Here's how the part is built. I have some questions about the finished solid (model axes, mm). A direction names the side the tool comes from. Round coordinates to 2 decimals unless told otherwise and drop trailing zeros. Write each loop counter-clockwise with the first axis right and the second up, starting at its lowest first coordinate (ties: lowest second). Pieces come first, ordered by that corner, then holes. Notation, with made-up numbers: (4.5, 50) - (35.5, 50) arc R15 cw to (35.5, 64) - close; hole circle Ø9 at (-3, 45). An arc over 180 degrees is marked (long way). Return JSON: item names as keys, results as strings. Group by question number.
```python
from build123d import *

# Parameters (mm, degrees)
SKETCH1_W               = 100
SKETCH1_H               = 45
BOSS_EXTRUDE1_DEPTH     = 90
CUT_EXTRUDE1_DEPTH      = 137.404728657
CUT_EXTRUDE2_DEPTH      = 109.397416943
CUT_EXTRUDE2_DEPTH_BACK = 109.397416943
SKETCH3_W               = 96
SKETCH3_H               = 32.638698082
SKETCH4_W               = 96
SKETCH4_H               = 35
CUT_EXTRUDE4_DEPTH      = 102.149641621
SKETCH5_R               = 8
SKETCH5_R_2             = 3
CUT_EXTRUDE5_DEPTH      = 134.158739856
SKETCH7_W               = 96
SKETCH7_H               = 3
CUT_EXTRUDE7_DEPTH      = 73.452349302
SKETCH9_W               = 50
SKETCH9_H               = 59.094844588
CUT_EXTRUDE9_DEPTH      = 34
SKETCH10_R              = 2
CUT_EXTRUDE10_DEPTH     = 34
CUT_EXTRUDE11_DEPTH     = 109.397416943
SKETCH11_W              = 96
SKETCH11_H              = 6.475085822
CUT_EXTRUDE12_DEPTH     = 34
SKETCH12_W              = 23
SKETCH12_H              = 26.924334535
CUT_EXTRUDE13_DEPTH     = 34


with BuildPart() as part:
    # Sketch1 → Boss-Extrude1 (new body)
    with BuildSketch(Plane.XY):
        Rectangle(SKETCH1_W, SKETCH1_H)
    extrude(amount=BOSS_EXTRUDE1_DEPTH)

    # Sketch2 → Cut-Extrude1 (cut, through all)
    with BuildSketch(Plane.ZY.offset(50)):
        Polygon((60, -22.5), (85, 20.5), (85, 22.5), (90, 22.5), (90, -22.5), align=None)
    extrude(amount=-CUT_EXTRUDE1_DEPTH, mode=Mode.SUBTRACT)

    # Sketch3 → Cut-Extrude2 (cut, two sides: drawn at the far end of the back side and taken through both)
    with BuildSketch(Plane(origin=(0, 22.5, 0), x_dir=(1, 0, 0), z_dir=(0, 1, 0)).offset(-CUT_EXTRUDE2_DEPTH_BACK)):
        with Locations((0, -21.319349041)):
            Rectangle(SKETCH3_W, SKETCH3_H)
    extrude(amount=CUT_EXTRUDE2_DEPTH + CUT_EXTRUDE2_DEPTH_BACK, mode=Mode.SUBTRACT)

    # Sketch4 → Cut-Extrude4 (cut, through all)
    with BuildSketch(Plane(origin=(0, 0, 0), x_dir=(-1, 0, 0), z_dir=(0, 0, -1))):
        Rectangle(SKETCH4_W, SKETCH4_H)
    extrude(amount=-CUT_EXTRUDE4_DEPTH, mode=Mode.SUBTRACT)

    # Sketch5 → Cut-Extrude5 (cut, through all)
    with BuildSketch(Plane(origin=(50, 0, 0), x_dir=(0, 0, -1), z_dir=(1, 0, 0))):
        with Locations(Location((-33, -3.5, 0), (0, 0, 90))):
            Circle(SKETCH5_R)
        with Locations(Location((-6.5, -3.5, 0), (0, 0, 90))):
            Circle(SKETCH5_R_2)
        with Locations(Location((-59.5, -3.5, 0), (0, 0, 90))):
            Circle(SKETCH5_R_2)
    extrude(amount=-CUT_EXTRUDE5_DEPTH, mode=Mode.SUBTRACT)

    # Sketch7 → Cut-Extrude7 (cut, through all)
    with BuildSketch(Plane(origin=(0, 0, 37.638698082), x_dir=(-1, 0, 0), z_dir=(0, 0, -1))):
        with Locations((0, 19)):
            Rectangle(SKETCH7_W, SKETCH7_H)
    extrude(amount=-CUT_EXTRUDE7_DEPTH, mode=Mode.SUBTRACT)

    # Sketch9 → Cut-Extrude9 (cut)
    with BuildSketch(Plane.XZ.offset(-20.5)):
        with Locations((0, 59.291541431)):
            Rectangle(SKETCH9_W, SKETCH9_H)
    extrude(amount=-CUT_EXTRUDE9_DEPTH, mode=Mode.SUBTRACT)

    # Sketch10 → Cut-Extrude10 (cut)
    with BuildSketch(Plane.XZ.offset(-20.5)):
        with Locations(Location((34.75, 78.05, 0), (0, 0, 270))):
            Circle(SKETCH10_R)
        with Locations(Location((34.75, 66.05, 0), (0, 0, 270))):
            Circle(SKETCH10_R)
        with Locations(Location((-34.75, 66.05, 0), (0, 0, 270))):
            Circle(SKETCH10_R)
        with Locations(Location((-34.75, 78.05, 0), (0, 0, 270))):
            Circle(SKETCH10_R)
    extrude(amount=-CUT_EXTRUDE10_DEPTH, mode=Mode.SUBTRACT)

    # Sketch8 → Cut-Extrude11 (cut, through all)
    with BuildSketch(Plane.XZ.offset(22.5)):
        Polygon((-48, 51.874077108), (-48, 37.638698082), (48, 37.638698082), (48, 51.874077108), (48, 55), (-48, 55), align=None)
    extrude(amount=-CUT_EXTRUDE11_DEPTH, mode=Mode.SUBTRACT)

    # Sketch11 → Cut-Extrude12 (cut)
    with BuildSketch(Plane.XZ.offset(22.5)):
        with Locations((0, 63.237542911)):
            Rectangle(SKETCH11_W, SKETCH11_H)
    extrude(amount=-CUT_EXTRUDE12_DEPTH, mode=Mode.SUBTRACT)

    # Sketch12 → Cut-Extrude13 (cut)
    with BuildSketch(Plane.XZ.offset(-20.5)):
        with Locations((-36.5, 46.537832733)):
            Rectangle(SKETCH12_W, SKETCH12_H)
        with Locations((36.5, 46.537832733)):
            Rectangle(SKETCH12_W, SKETCH12_H)
    extrude(amount=-CUT_EXTRUDE13_DEPTH, mode=Mode.SUBTRACT)


solid = part.part
```
1) Imagine slicing it at C-C (x = -21). Please give me the cut outline in (y, z).
2) For faces 5 (the flat face through (-1, -20, 5)), 6 (the cylindrical face through (49.01, -4.15, 3.57)), 7 (the flat face through (-1, -20, 60)), 8 (the flat face through (-49.014, -1.301, 72.325)), 9 (the flat face through (1, -17.5, 2)), which set-ups out of +Z, -Z, +X, -X, +Y, -Y let a thin tool reach every point of the face, with its end or its side?
3) Imagine slicing it at A-A (x = 30). Please give me the cut outline in (y, z).
4) If we mould it in two halves opening along Y, with no side actions, what happens to faces 1 (the flat face through (1, 17.5, 2)), 2 (the flat face through (37, 20.5, 72)), 3 (the flat face through (1, -17.5, 57)), 4 (the cylindrical face through (49.014, -4.541, 40.932))? For each: released by +Y, released by -Y, zero draft, split by the parting line, or undercut.
5) I need wall thicknesses on line 1 along X through (y, z) = (21.4, 66.05); line 2 along X through (y, z) = (-12, 19); line 3 along Z through (x, y) = (-48.5, -3.5). Which ranges of each line are inside material? Lowest first, please.
6) Will these pins go through, and if not, where does the flat tip stop? pin 1 Ø7 at (x, z) = (34.5, 70.5) entering from -Y; pin 2 Ø5.5 at (y, z) = (-3.5, 59.5) entering from +X; pin 3 Ø2.5 at (x, y) = (20.5, -20) entering from +Z; pin 4 Ø5.5 at (x, y) = (-2.5, 20.5) entering from +Z.
7) Imagine slicing it at B-B (z = 33). Please give me the cut outline in (x, y), plus the area to 3 significant figures.
8) Imagine slicing it at D-D (z = 20). Please give me the cut outline in (x, y).
Results found:
{
 "1": {"outline": "(-22.5, 0) - (-17.5, 0) - (-17.5, 5) - (-22.5, 5) - close; (-22.5, 55) - (-17.5, 55) - (-17.5, 60) - (-22.5, 60) - close; (17.5, 0) - (22.5, 0) - (22.5, 5) - (17.5, 5) - close"},
 "2": {"face 5": "+Y, -Y", "face 6": "+X, -X", "face 7": "+Z, -Y", "face 8": "+Z, +X, -X, -Y", "face 9": "+Z, -Z"},
 "3": {"outline": "(-22.5, 0) - (-17.5, 0) - (-17.5, 5) - (-22.5, 5) - close; (-22.5, 55) - (-17.5, 55) - (-17.5, 60) - (-22.5, 60) - close; (17.5, 0) - (22.5, 0) - (22.5, 5) - (17.5, 5) - close; (20.5, 60) - (22.5, 60) - (22.5, 85) - (20.5, 85) - close"},
 "4": {"face 1": "undercut", "face 2": "released by -Y", "face 3": "released by +Y", "face 4": "undercut"},
 "5": {"line 1": "x = -50 to -36.75, -32.75 to -25, 25 to 32.75, 36.75 to 50", "line 2": "x = -50 to -48, 48 to 50", "line 3": "z = 0 to 3.5, 9.5 to 25, 41 to 56.5, 62.5 to 71.05"},
 "6": {"pin 1": "stops at y = 20.5", "pin 2": "passes through", "pin 3": "stops at z = 60", "pin 4": "stops at z = 5"},
 "7": {"outline": "(-50, -22.5) - (-48, -22.5) - (-48, -11.5) - (-50, -11.5) - close; (-50, 4.5) - (-48, 4.5) - (-48, 22.5) - (-50, 22.5) - close; (48, -22.5) - (50, -22.5) - (50, -11.5) - (48, -11.5) - close; (48, 4.5) - (50, 4.5) - (50, 22.5) - (48, 22.5) - close", "area": "116 mm²"},
 "8": {"outline": "(-50, -22.5) - (-48, -22.5) - (-48, 22.5) - (-50, 22.5) - close; (48, -22.5) - (50, -22.5) - (50, 22.5) - (48, 22.5) - close"}
}
